Design review of the part built by this model. Coordinates are the model's own, in mm. Face numbers are marked on the shaded views. A direction names the side the tool comes from. Round coordinates to 2 decimals unless told otherwise and drop trailing zeros. Loops run counter-clockwise (first coordinate to the right, second up) from the corner with the lowest first, then second, coordinate; pieces in that order, holes last. Notation, with made-up numbers: M 44.5,9 L 85.5,9 A19 ccw 85.5,35 Z; hole C 25.25,8.25 d9. An arc over 180 degrees is marked long. One line per item, written item: value. Start each with the question number.
Item 1: We need section A-A (x = 24.5). Write out the cut boundary in (y, z).
Item 2: For line 1 along Y through (x, z) = (25, 6.5); line 2 along X through (y, z) = (5.5, 26.5), list the stretches that pass through material, from the lowest coordinate up.
Item 3: For the marked faces 1 and 2, list the 3-axis set-ups (+Z, -Z, +X, -X, +Y, -Y) from which the entire face can be reached by the end or side of a thin tool; tool diameter is ignored.
Item 4: We need section B-B (y = 21.25). Write out the cut boundary in (x, z), then the cut area to 3 significant figures.
Item 5: We need section D-D (z = 28.5). Write out the cut boundary in (x, y), then the cut area to 3 significant figures.
Item 6: We need section C-C (y = 18). Write out the cut boundary in (x, z), then the cut area to 3 significant figures.
Item 7: Clearance check with flat-ended pins moving along their axes: pin 1 (2 mm diameter, centred on x = 24, y = 19.5, fed in from -Z); pin 2 (1 mm diameter, centred on y = 15, z = 9, fed in from +X); pin 3 (5 mm diameter, centred on x = 26.5, z = 23, fed in from -Y); pin 4 (1.5 mm diameter, centred on x = 26.5, y = 15.5, fed in from +Z). State where each tip first meets the part, or that it passes through.
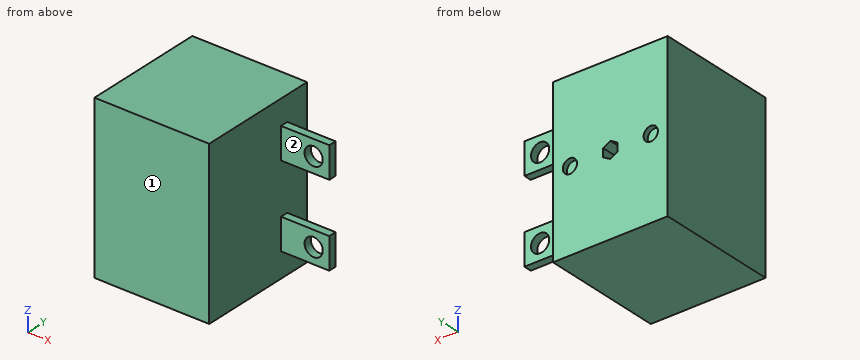
from build123d import *

# Parameters (mm, degrees)
SKETCH1_W           = 22.352
SKETCH1_H           = 23.876
BOSS_EXTRUDE1_DEPTH = 31.75
CUT_EXTRUDE1_DEPTH  = 4.572
SKETCH2_3_R         = 1.3890625
CUT_EXTRUDE2_DEPTH  = 1
SKETCH4_W           = 6.096
SKETCH4_H           = 1.524
BOSS_EXTRUDE2_DEPTH = 9.398
CUT_EXTRUDE3_REACH  = 50.775
SKETCH5_R           = 1.778


with BuildPart() as part:
    # Sketch1 → Boss-Extrude1 (new body)
    with BuildSketch(Plane.XY):
        with Locations((11.176, 11.938)):
            Rectangle(SKETCH1_W, SKETCH1_H)
    extrude(amount=BOSS_EXTRUDE1_DEPTH)

    # Sketch2 → Cut-Extrude1 (cut)
    with BuildSketch(Plane(origin=(0, 23.876, 0), x_dir=(1, 0, 0), z_dir=(0, 1, 0))):
        Polygon((9.7869375, -14.946024392), (9.7869375, -16.549975608), (11.176, -17.351951217), (12.5650625, -16.549975608), (12.5650625, -14.946024392), (11.176, -14.144048783), align=None)
    extrude(amount=-CUT_EXTRUDE1_DEPTH, mode=Mode.SUBTRACT)

    # Sketch2_3 → Cut-Extrude2 (cut)
    with BuildSketch(Plane(origin=(0, 23.876, 0), x_dir=(1, 0, 0), z_dir=(0, 1, 0))):
        with Locations(Location((19.05, -15.748, 0), (0, 0, 270))):
            Circle(SKETCH2_3_R)
        with Locations(Location((3.302, -15.748, 0), (0, 0, 270))):
            Circle(SKETCH2_3_R)
    extrude(amount=-CUT_EXTRUDE2_DEPTH, mode=Mode.SUBTRACT)

    # Sketch4 → Boss-Extrude2 (add)
    with BuildSketch(Plane(origin=(22.352, 0, 0), x_dir=(0, 0, -1), z_dir=(1, 0, 0))):
        with Locations((-23.876, 18.288)):
            Rectangle(SKETCH4_W, SKETCH4_H)
        with Locations((-7.874, 18.288)):
            Rectangle(SKETCH4_W, SKETCH4_H)
    extrude(amount=BOSS_EXTRUDE2_DEPTH)

    # Sketch5 → Cut-Extrude3 (cut, up to next)
    with BuildSketch(Plane(origin=(0, 19.05, 0), x_dir=(1, 0, 0), z_dir=(0, 1, 0)), mode=Mode.PRIVATE) as cut_extrude3_sk1:
        with Locations(Location((28.702, -23.876, 0), (0, 0, 180))):
            Circle(SKETCH5_R)
    cut_extrude3_tool1 = extrude(cut_extrude3_sk1.sketch, amount=-CUT_EXTRUDE3_REACH, mode=Mode.PRIVATE) & part.part
    # Sketch5 → Cut-Extrude3 (cut, up to next)
    with BuildSketch(Plane(origin=(0, 19.05, 0), x_dir=(1, 0, 0), z_dir=(0, 1, 0)), mode=Mode.PRIVATE) as cut_extrude3_sk2:
        with Locations(Location((28.702, -7.874, 0), (0, 0, 180))):
            Circle(SKETCH5_R)
    cut_extrude3_tool2 = extrude(cut_extrude3_sk2.sketch, amount=-CUT_EXTRUDE3_REACH, mode=Mode.PRIVATE) & part.part
    add(cut_extrude3_tool1.solids().sort_by_distance((28.702, 19.05, 23.876))[0], mode=Mode.SUBTRACT)
    add(cut_extrude3_tool2.solids().sort_by_distance((28.702, 19.05, 7.874))[0], mode=Mode.SUBTRACT)


solid = part.part
A:
1. outline: M 17.53,4.83 L 19.05,4.83 L 19.05,10.92 L 17.53,10.92 Z; M 17.53,20.83 L 19.05,20.83 L 19.05,26.92 L 17.53,26.92 Z
2. line 1: 17.53 to 19.05
2. line 2: 0 to 22.35
3. face 1: +Z, -Z, +X, -X, -Y
3. face 2: +Z, -Z, +X, -Y
4. outline: M 0,0 L 22.35,0 L 22.35,31.75 L 0,31.75 Z; hole M 9.79,14.95 L 11.18,14.14 L 12.57,14.95 L 12.57,16.55 L 11.18,17.35 L 9.79,16.55 Z
4. area: 703 mm2
5. outline: M 0,0 L 22.35,0 L 22.35,23.88 L 0,23.88 Z
5. area: 534 mm2
6. outline: M 0,0 L 22.35,0 L 22.35,4.83 L 31.75,4.83 L 31.75,10.92 L 22.35,10.92 L 22.35,20.83 L 31.75,20.83 L 31.75,26.92 L 22.35,26.92 L 22.35,31.75 L 0,31.75 Z; hole C 28.7,7.87 d3.56; hole C 28.7,23.88 d3.56
6. area: 804 mm2
7. pin 1: z = 4.83
7. pin 2: x = 22.35
7. pin 3: y = 17.53
7. pin 4: through
